Model file for the job. Use its own axes, mm. A direction names the side the tool comes from. Round coordinates to 2 decimals unless told otherwise and drop trailing zeros. Loops run counter-clockwise (first coordinate to the right, second up) from the corner with the lowest first, then second, coordinate; pieces in that order, holes last. Notation, with made-up numbers: M -7.75,-3.75 L 36.25,-3.75 A9 ccw 36.25,12.25 Z; hole C 36.25,31 d2. An arc over 180 degrees is marked long. Answer in a Markdown table with one row per item.
from build123d import *

# Parameters (mm, degrees)
CIRPATTERN1_COUNT        = 3
CHAMFER1_SIZE            = 0.5
CHAMFER2_SIZE            = 1
CUT_EXTRUDE1_DEPTH       = 51.319429647
FILLET1_R                = 1.5
M3X0_5_TAPPED_HOLE1_D    = 2.5
CIRPATTERN2_COUNT        = 6
FILLET1_OF_CIRPATTERN2_R = 1.5
SKETCH10_W               = 1.207732619
SKETCH10_H               = 1.1
SKETCH11_W               = 3.151954219
SKETCH11_H               = 1.1
M3X0_5_TAPPED_HOLE2_D    = 2.5
CIRPATTERN3_COUNT        = 6
CHAMFER3_SIZE            = 0.5


with BuildPart() as part:
    # Sketch2 → Revolve1 (revolve)
    with BuildSketch(Plane.XY, mode=Mode.PRIVATE) as revolve1_sk:
        Polygon((-4, 10), (-4, -6.5), (-3.1, -6.5), (-3.1, -9.5), (-4.1, -9.5), (-4.1, -7.5), (-6, -7.5), (-6, 10), (-7, 10), (-7, 17), (-32.65, 17), (-32.65, 20), (-5, 20), (-5, 11), align=None)
    revolve(revolve1_sk.sketch.rotate(Axis((0, 0, 0), (0, -1, 0)), 270), axis=Axis((0, 0, 0), (0, -1, 0)))

    # Sketch3 → Revolve2 (revolve)
    with BuildSketch(Plane.XY):
        Polygon((-21.598, 15), (-22.598, 15), (-22.598, 17), (-20.098, 17), (-20.098, 11), (-21.598, 11), align=None)
    revolve2 = revolve(axis=Axis((-20.098, 18.273035546, 0), (0, -1, 0)))

    # CirPattern1: Revolve2 ×3 about axis
    cirpattern1_axis = Axis((0, 0, 0), (0, 1, 0))
    for i in range(1, CIRPATTERN1_COUNT):
        add(revolve2.rotate(cirpattern1_axis, i * 360 / CIRPATTERN1_COUNT))

    # Chamfer1
    chamfer1_edges = [part.edges().sort_by_distance(p)[0] for p in [
        (0, 20, -32.65),
        (0, 17, -32.65),
    ]]
    chamfer(chamfer1_edges, length=CHAMFER1_SIZE)

    # Chamfer2
    chamfer2_edges = [part.edges().sort_by_distance(p)[0] for p in [
        (0, 20, -5),
    ]]
    chamfer(chamfer2_edges, length=CHAMFER2_SIZE)

    # Sketch6 → Cut-Extrude1 (cut, through all)
    with BuildSketch(Plane(origin=(0, 0, 0), x_dir=(1, 0, 0), z_dir=(0, 1, 0))):
        with BuildLine():
            Line((24.899246977, -9.5), (10.95445115, -1))
            ThreePointArc((10.95445115, -1), (11, 0), (10.95445115, 1))
            Line((10.95445115, 1), (24.899246977, 9.5))
            ThreePointArc((24.899246977, 9.5), (26.65, 0), (24.899246977, -9.5))
        make_face()
    cut_extrude1 = extrude(amount=CUT_EXTRUDE1_DEPTH, mode=Mode.SUBTRACT)

    # Fillet1
    fillet1_edges = [part.edges().sort_by_distance(p)[0] for p in [
        (24.899246977, 18.5, 9.5),
        (24.899246977, 18.5, -9.5),
        (10.95445115, 18.5, -1),
        (10.95445115, 18.5, 1),
    ]]
    fillet(fillet1_edges, radius=FILLET1_R)

    # M3x0.5 Tapped Hole1 (through all)
    with Locations(Plane(origin=(0, 20, 0), x_dir=(1, 0, 0), z_dir=(0, 1, 0))):
        with Locations((12.990381057, -7.5)):
            m3x0_5_tapped_hole1 = Hole(M3X0_5_TAPPED_HOLE1_D / 2)

    # CirPattern2: Cut-Extrude1, M3x0.5 Tapped Hole1 ×6 about axis
    cirpattern2_axis = Axis((0, 0, 0), (0, 1, 0))
    add([cut_extrude1.rotate(cirpattern2_axis, i * 360 / CIRPATTERN2_COUNT) for i in range(1, CIRPATTERN2_COUNT)], mode=Mode.SUBTRACT)
    add([m3x0_5_tapped_hole1.rotate(cirpattern2_axis, i * 360 / CIRPATTERN2_COUNT) for i in range(1, CIRPATTERN2_COUNT)], mode=Mode.SUBTRACT)

    # Fillet1 of CirPattern2
    fillet1_of_cirpattern2_edges = [part.edges().sort_by_distance(p)[0] for p in [
        (20.676864824, 18.5, -16.813380417),
        (4.222382152, 18.5, -26.313380417),
        (4.611200171, 18.5, -9.986832981),
        (6.343250979, 18.5, -8.986832981),
        (-4.222382152, 18.5, -26.313380417),
        (-20.676864824, 18.5, -16.813380417),
        (-6.343250979, 18.5, -8.986832981),
        (-4.611200171, 18.5, -9.986832981),
        (-24.899246977, 18.5, -9.5),
        (-24.899246977, 18.5, 9.5),
        (-10.95445115, 18.5, 1),
        (-10.95445115, 18.5, -1),
        (-20.676864824, 18.5, 16.813380417),
        (-4.222382152, 18.5, 26.313380417),
        (-4.611200171, 18.5, 9.986832981),
        (-6.343250979, 18.5, 8.986832981),
        (4.222382152, 18.5, 26.313380417),
        (20.676864824, 18.5, 16.813380417),
        (6.343250979, 18.5, 8.986832981),
        (4.611200171, 18.5, 9.986832981),
    ]]
    fillet(fillet1_of_cirpattern2_edges, radius=FILLET1_OF_CIRPATTERN2_R)

    # Sketch9 → Cut-Revolve1 (revolve, cut)
    with BuildSketch(Plane.XY, mode=Mode.PRIVATE) as cut_revolve1_sk:
        Polygon((-8.538708616, -5.4), (-5.75, -5.4), (-5.75, -6.5), (-6.5, -6.5), (-5.5, -7.5), (-8.538708616, -7.5), align=None)
    revolve(cut_revolve1_sk.sketch.rotate(Axis((0, 0, 0), (0, -1, 0)), 270), axis=Axis((0, 0, 0), (0, -1, 0)), mode=Mode.SUBTRACT)

    # Sketch10 → Cut-Revolve2 (revolve, cut)
    with BuildSketch(Plane.XY, mode=Mode.PRIVATE) as cut_revolve2_sk:
        with Locations((-6.35386631, 5.45)):
            Rectangle(SKETCH10_W, SKETCH10_H)
    revolve(cut_revolve2_sk.sketch.rotate(Axis((0, 0, 0), (0, 1, 0)), 90), axis=Axis((0, 0, 0), (0, 1, 0)), mode=Mode.SUBTRACT)

    # Sketch11 → Cut-Revolve3 (revolve, cut)
    with BuildSketch(Plane.XY, mode=Mode.PRIVATE) as cut_revolve3_sk:
        with Locations((-7.32597711, 3.15)):
            Rectangle(SKETCH11_W, SKETCH11_H)
    revolve(cut_revolve3_sk.sketch.rotate(Axis((0, 0, 0), (0, -1, 0)), 270), axis=Axis((0, 0, 0), (0, -1, 0)), mode=Mode.SUBTRACT)

    # M3x0.5 Tapped Hole2 (through all)
    with Locations(Plane(origin=(0, 20, 0), x_dir=(1, 0, 0), z_dir=(0, 1, 0))):
        with Locations((0, 30)):
            m3x0_5_tapped_hole2 = Hole(M3X0_5_TAPPED_HOLE2_D / 2)

    # CirPattern3: M3x0.5 Tapped Hole2 ×6 about axis
    cirpattern3_axis = Axis((0, 0, 0), (0, 1, 0))
    for i in range(1, CIRPATTERN3_COUNT):
        add(m3x0_5_tapped_hole2.rotate(cirpattern3_axis, i * 360 / CIRPATTERN3_COUNT), mode=Mode.SUBTRACT)

    # Chamfer3
    chamfer3_edges = [part.edges().sort_by_distance(p)[0] for p in [
        (13.081967435, 20, -12.666357528),
        (13.325, 20, -23.079577011),
        (5.5, 20, -9.526279442),
        (4.428403676, 20, -17.662494894),
        (19.798373681, 20, -16.997842711),
        (6.380220105, 20, -9.232137893),
        (4.805155894, 20, -10.141501639),
        (4.821376756, 20, -25.644815917),
        (-4.428403676, 20, -17.662494894),
        (-13.325, 20, -23.079577011),
        (-5.5, 20, -9.526279442),
        (-13.081967435, 20, -12.666357528),
        (-4.821376756, 20, -25.644815917),
        (-4.805155894, 20, -10.141501639),
        (-6.380220105, 20, -9.232137893),
        (-19.798373681, 20, -16.997842711),
        (-17.51037111, 20, -4.996137366),
        (-26.65, 20, 0),
        (-11, 20, 0),
        (-17.51037111, 20, 4.996137366),
        (-24.619750438, 20, -8.646973206),
        (-11.185375999, 20, -0.909363746),
        (-11.185375999, 20, 0.909363746),
        (-24.619750438, 20, 8.646973206),
        (-13.081967435, 20, 12.666357528),
        (-13.325, 20, 23.079577011),
        (-5.5, 20, 9.526279442),
        (-4.428403676, 20, 17.662494894),
        (-19.798373681, 20, 16.997842711),
        (-6.380220105, 20, 9.232137893),
        (-4.805155894, 20, 10.141501639),
        (-4.821376756, 20, 25.644815917),
        (4.428403676, 20, 17.662494894),
        (13.325, 20, 23.079577011),
        (5.5, 20, 9.526279442),
        (13.081967435, 20, 12.666357528),
        (4.821376756, 20, 25.644815917),
        (4.805155894, 20, 10.141501639),
        (6.380220105, 20, 9.232137893),
        (19.798373681, 20, 16.997842711),
        (17.51037111, 20, 4.996137366),
        (26.65, 20, 0),
        (11, 20, 0),
        (17.51037111, 20, -4.996137366),
        (24.619750438, 20, 8.646973206),
        (11.185375999, 20, 0.909363746),
        (11.185375999, 20, -0.909363746),
        (24.619750438, 20, -8.646973206),
    ]]
    chamfer(chamfer3_edges, length=CHAMFER3_SIZE)


solid = part.part
1. Wall check: probe 1 along Z at (x, y) = (18, 19.25); probe 2 along X at (y, z) = (17.75, -14); probe 3 along Y at (x, z) = (6.5, 3.5). Give the ranges that are in metal, low to high.
Verdict:
| item | result |
|---|---|
| probe 1 | z = -27.24 to -19.65, -15.35 to -5.29, 5.29 to 15.35, 19.65 to 27.24 |
| probe 2 | x = -29.5 to -26.73, -25.23 to -15.52, -4.52 to -0.75, 0.75 to 4.52, 15.52 to 25.23, 26.73 to 29.5 |
| probe 3 | y = 17 to 20 |
2. Pin check, flat tips, straight feed: pin 1 (4 mm diameter, centred on x = -4.5, z = -9.5, fed in from -Y); pin 2 (6 mm diameter, centred on y = 15.5, z = 24.5, fed in from +X); pin 3 (1.5 mm diameter, centred on x = 0.5, y = 6, fed in from -Z). Stop position of each tip, or through.
Verdict:
| item | result |
|---|---|
| pin 1 | stops at y = 17 |
| pin 2 | stops at x = 23.88 |
| pin 3 | stops at z = -6 |
3. Tool access for faces 4 (the flat face through (-13.283, 19.746, 12.496)), 5 (the cylindrical face through (6.834, 13.549, -1.517)), 6 (the cylindrical face through (24.602, 18.268, -8.654)), 7 (the cylindrical face through (-4.85, -5.96, 3.09)): list every direction of +Z, -Z, +X, -X, +Y, -Y with a clear straight run to the whole face (end or side of a thin tool).
Verdict:
| item | result |
|---|---|
| face 4 | +Y |
| face 5 | -Y |
| face 6 | +Y, -Y |
| face 7 | none |
4. Saw through at B-B (z = -21.5). State how many separate pieces and enclosed holes the cut face has, and give its area (3 significant figures).
Verdict:
| item | result |
|---|---|
| separate pieces | 3 |
| enclosed holes | 0 |
| area | 77.6 mm² |
5. Mould opens along Z. For faces 1 (the flat face through (7, 17, -7)), 2 (the cylindrical face through (19.8, 18.3, 17)), 3 (the cylindrical face through (-1.802, -1.344, 5.723)) say: +Z half, -Z half, draft (parallel to the pull), parting line (faces both ways), or undercut.
Verdict:
| item | result |
|---|---|
| face 1 | draft |
| face 2 | undercut |
| face 3 | parting line |
6. Saw through at A-A (y = -0.25). Write the cut outline in (x, z).
Verdict:
| item | result |
|---|---|
| outline | C 0,0 d12; hole C 0,0 d8 |
